from build123d import *

# Parameters (mm, degrees)
ROTATION1_ANGLE                                     = 180
SCHNITT_LINEAR_AUSTRAGEN2_DEPTH                     = 92.33454987
SCHNITT_LINEAR_AUSTRAGEN2_DEPTH_BACK                = 90
SCHNITT_LINEAR_AUSTRAGEN3_DEPTH                     = 92.33454987
SCHNITT_LINEAR_AUSTRAGEN3_DEPTH_BACK                = 90
SKIZZE8_W                                           = 10
SKIZZE8_H                                           = 5
AUFSATZ_LINEAR_AUSTRAGEN2_DEPTH                     = 90
SKIZZE9_W                                           = 10
SKIZZE9_H                                           = 5
AUFSATZ_LINEAR_AUSTRAGEN3_DEPTH                     = 90
SKIZZE16_R                                          = 1.1
SCHNITT_LINEAR_AUSTRAGEN8_DEPTH                     = 93.717898057
SKIZZE18_R                                          = 4
SCHNITT_LINEAR_AUSTRAGEN9_DEPTH                     = 5
SKIZZE20_W                                          = 21.700648505
SKIZZE20_H                                          = 2
SCHNITT_LINEAR_AUSTRAGEN10_DEPTH                    = 93.717898057
SKIZZE22_R                                          = 11.608493419
SKIZZE22_R_2                                        = 11.500591483
SCHNITT_LINEAR_AUSTRAGEN17_DEPTH                    = 93.501938467
SKIZZE24_W                                          = 4
SKIZZE24_H                                          = 5
SCHNITT_LINEAR_AUSTRAGEN18_DEPTH                    = 93.501938467
STIRNSENKUNG_F_R_M2_SECHSKANTSCHRAUBE_G_D           = 2.2
STIRNSENKUNG_F_R_M2_SECHSKANTSCHRAUBE_G_DEPTH       = 12
STIRNSENKUNG_F_R_M2_SECHSKANTSCHRAUBE_G_CBORE_D     = 6.38
STIRNSENKUNG_F_R_M2_SECHSKANTSCHRAUBE_G_CBORE_DEPTH = 3.1
STIRNSENKUNG_F_R_M2_SECHSKANTSCHRAUBE_G_TIP         = 0.660946681


with BuildPart() as part:
    # Skizze3 → Rotation1 (revolve)
    with BuildSketch(Plane.XY):
        Polygon((0, 0), (-11, 0), (-11, 90), (-6, 90), (-6, 10), (0, 10), align=None)
    revolve(axis=Axis((0, 0, 0), (0, 1, 0)), revolution_arc=ROTATION1_ANGLE)

    # Skizze6 → Schnitt-Linear austragen2 (cut, two sides: drawn at the far end of the back side and taken through both)
    with BuildSketch(Plane(origin=(0, 90, 0), x_dir=(1, 0, 0), z_dir=(0, 1, 0)).offset(-SCHNITT_LINEAR_AUSTRAGEN2_DEPTH_BACK)):
        Polygon((-9.380624863, -62.0642209), (-9.380624863, -5.744900102), (-9.380624863, 0), (-9.380624863, 56.319320799), (-122.01926646, 56.319320799), (-122.01926646, -62.0642209), align=None)
    extrude(amount=SCHNITT_LINEAR_AUSTRAGEN2_DEPTH + SCHNITT_LINEAR_AUSTRAGEN2_DEPTH_BACK, mode=Mode.SUBTRACT)

    # Skizze7 → Schnitt-Linear austragen3 (cut, two sides: drawn at the far end of the back side and taken through both)
    with BuildSketch(Plane.XZ.offset(-SCHNITT_LINEAR_AUSTRAGEN3_DEPTH_BACK)):
        Polygon((9.380624863, 59.241313346), (9.380624863, 5.744900102), (9.380624863, 0), (9.380624863, -53.496413245), (116.373451353, -53.496413245), (116.373451353, 59.241313346), align=None)
    extrude(amount=SCHNITT_LINEAR_AUSTRAGEN3_DEPTH + SCHNITT_LINEAR_AUSTRAGEN3_DEPTH_BACK, mode=Mode.SUBTRACT)

    # Skizze8 → Aufsatz-Linear austragen2 (add)
    with BuildSketch(Plane(origin=(0, 90, 0), x_dir=(1, 0, 0), z_dir=(0, 1, 0))):
        with Locations((-14.380624863, -2.5)):
            Rectangle(SKIZZE8_W, SKIZZE8_H)
    extrude(amount=-AUFSATZ_LINEAR_AUSTRAGEN2_DEPTH)

    # Skizze9 → Aufsatz-Linear austragen3 (add)
    with BuildSketch(Plane(origin=(0, 90, 0), x_dir=(1, 0, 0), z_dir=(0, 1, 0))):
        with Locations((14.380624863, -2.5)):
            Rectangle(SKIZZE9_W, SKIZZE9_H)
    extrude(amount=-AUFSATZ_LINEAR_AUSTRAGEN3_DEPTH)

    # Skizze16 → Schnitt-Linear austragen8 (cut, through all)
    with BuildSketch(Plane.XZ):
        Circle(SKIZZE16_R)
    extrude(amount=-SCHNITT_LINEAR_AUSTRAGEN8_DEPTH, mode=Mode.SUBTRACT)

    # Skizze18 → Schnitt-Linear austragen9 (cut)
    with BuildSketch(Plane.XZ):
        Circle(SKIZZE18_R)
    extrude(amount=-SCHNITT_LINEAR_AUSTRAGEN9_DEPTH, mode=Mode.SUBTRACT)

    # Skizze20 → Schnitt-Linear austragen10 (cut, through all)
    with BuildSketch(Plane(origin=(0, 90, 0), x_dir=(1, 0, 0), z_dir=(0, 1, 0))):
        with Locations((-0.450220923, -10)):
            Rectangle(SKIZZE20_W, SKIZZE20_H)
    extrude(amount=-SCHNITT_LINEAR_AUSTRAGEN10_DEPTH, mode=Mode.SUBTRACT)

    # Skizze22 → Schnitt-Linear austragen17 (cut, through all)
    with BuildSketch(Plane(origin=(0, 90, 0), x_dir=(1, 0, 0), z_dir=(0, 1, 0))):
        with Locations((-14.380624863, -15.356814397)):
            Circle(SKIZZE22_R)
        with Locations((14.380624863, -15.356814397)):
            Circle(SKIZZE22_R_2)
    extrude(amount=-SCHNITT_LINEAR_AUSTRAGEN17_DEPTH, mode=Mode.SUBTRACT)

    # Skizze24 → Schnitt-Linear austragen18 (cut, through all)
    with BuildSketch(Plane(origin=(0, 90, 0), x_dir=(1, 0, 0), z_dir=(0, 1, 0))):
        with Locations((17.380624863, -2.5)):
            Rectangle(SKIZZE24_W, SKIZZE24_H)
        with Locations((-17.380624863, -2.5)):
            Rectangle(SKIZZE24_W, SKIZZE24_H)
    extrude(amount=-SCHNITT_LINEAR_AUSTRAGEN18_DEPTH, mode=Mode.SUBTRACT)

    # Stirnsenkung für M2 Sechskantschraube, Gewinde bis Kopf10
    with Locations(Plane(origin=(-0.023013558, 0, 6.13421813), x_dir=(-0.9999929625632231, 0, -0.0037516428439037797), z_dir=(-0.0037516428439037797, 0, 0.9999929625632231))):
        with Locations((11.36629237, -82), (11.36629237, -8), (-11.39514721, -8), (-11.39514721, -82)):
            CounterBoreHole(STIRNSENKUNG_F_R_M2_SECHSKANTSCHRAUBE_G_D / 2, STIRNSENKUNG_F_R_M2_SECHSKANTSCHRAUBE_G_CBORE_D / 2, STIRNSENKUNG_F_R_M2_SECHSKANTSCHRAUBE_G_CBORE_DEPTH, depth=STIRNSENKUNG_F_R_M2_SECHSKANTSCHRAUBE_G_DEPTH)
            with Locations((0, 0, -(STIRNSENKUNG_F_R_M2_SECHSKANTSCHRAUBE_G_DEPTH + STIRNSENKUNG_F_R_M2_SECHSKANTSCHRAUBE_G_TIP / 2))):  # 118° drill point
                Cone(0, STIRNSENKUNG_F_R_M2_SECHSKANTSCHRAUBE_G_D / 2, STIRNSENKUNG_F_R_M2_SECHSKANTSCHRAUBE_G_TIP, mode=Mode.SUBTRACT)


solid = part.part
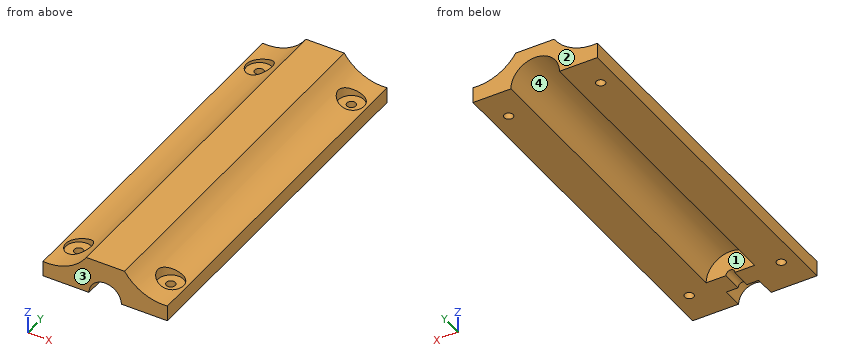
Check sheet for the modelled part. Datum: model origin and axes. Units: mm. Face numbers are marked on the shaded views. A direction names the side the tool comes from. Give positions to 0.01 mm unless a question says otherwise; leave off trailing zeros. Loops run counter-clockwise (first coordinate to the right, second up) from the corner with the lowest first, then second, coordinate; pieces in that order, holes last. Notation, with made-up numbers: M 77.5,16 L 131.5,16 A12 cw 131.5,39 Z; hole C 2.5,44 d8. An arc over 180 degrees is marked long. Answer as a JSON object with one key per item and string values. Group by question number.
Q1. Cross-section at C-C on z = 8. Record the cut outline in (x, y), then the cut area to 3 significant figures.
Q2. Cross-section at B-B on y = 65. Record the cut outline in (x, z), then the cut area to 3 significant figures.
Q3. Cross-section at D-D on x = 7. Record the cut outline in (y, z).
Q4. Go/stop test with flat-tipped pins: P1, Ø6, axis at x = -2, y = 38, coming from the -Z side; P2, Ø8, axis at x = -9, y = 49, coming from the +Z side; P3, Ø3, axis at y = 60, z = 7.5, coming from the +X side; P4, Ø3, axis at x = -4, z = 1.5, coming from the -Y side. Record where each tip stops, or that it passes through.
Q5. Material ranges on line 1 along Y through (x, z) = (-11.5, 3.5); line 2 along Y through (x, z) = (5, 0.75); line 3 along Y through (x, z) = (-1, 2.25), recorded low to high. Write a range as [from, to].
Q6. Cross-section at A-A on x = 0. Record the cut outline in (y, z), then the cut area to 4 significant figures.
Q7. Access from +Z, -Z, +X, -X, +Y, -Y to the whole of each face (thin tool, end or side, straight path). Record for the marked faces 3 and 4.
Q8. Release check for a two-part mould opening along X. For the marked faces 1 and 2 record: released by +X, released by -X, zero draft, split by the parting line, or undercut.
Evaluation:
{
 "1": {"outline": "M -5.4,0 L 5.54,0 L 5.54,90 L -5.4,90 Z", "area": "985 mm2"},
 "2": {"outline": "M -15.38,0 L -6,0 A6 cw 6,0 L 15.38,0 L 15.38,3.9 A11.5 cw 4.8,9 L -4.67,9 A11.61 cw -15.38,3.79 Z", "area": "139 mm2"},
 "3": {"outline": "M 0,0 L 90,0 L 90,6.54 L 0,6.54 Z"},
 "4": {"P1": "stops at z = 3.32", "P2": "stops at z = 8.52", "P3": "stops at x = 7.69", "P4": "stops at y = 0"},
 "5": {"line 1": "y = [0, 4.81], [11.19, 78.81], [85.19, 90]", "line 2": "y = [0, 10]", "line 3": "y = [5, 10]"},
 "6": {"outline": "M 0,4 L 5,4 L 5,1.1 L 10,1.1 L 10,6 L 90,6 L 90,9 L 0,9 Z", "area": "304.5 mm2"},
 "7": {"face 3": "+Z, -Z, +X, -X, -Y", "face 4": "-Z, +Y"},
 "8": {"face 1": "undercut", "face 2": "zero draft"}
}
